Answer from the drawing. Dimensions are ordinates in mm from the lowest x, y and z of the part. Coordinates: 2 decimals unless noted, no trailing zeros. Loops run counter-clockwise (first coordinate to the right, second up) from the corner with the lowest first, then second, coordinate; pieces in that order, holes last. Notation, with made-up numbers: (60.25, 32) -> (92.25, 32) arc R10 ccw to (92.25, 41) -> close; hole circle Ø3 at (6.5, 67). An arc over 180 degrees is marked (long way). Answer as CSV lines item,"result".
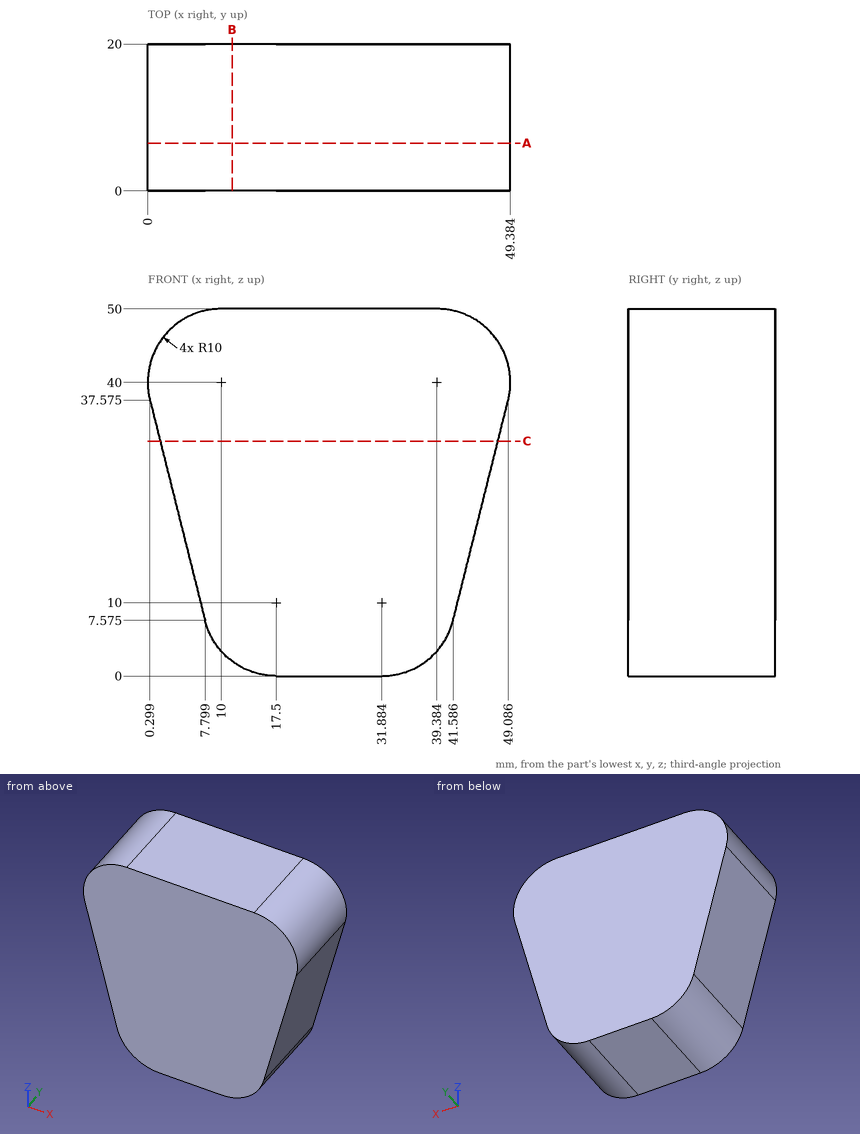
(1) A cutting plane is placed at A-A, the plane y = 6.5. Write down the section's boundary in (x, z) (1 decimal).
Computed values:
outline,"(0.3, 37.6) -> (7.8, 7.6) arc R10 ccw to (17.5, 0) -> (31.9, 0) arc R10 ccw to (41.6, 7.6) -> (49.1, 37.6) arc R10 ccw to (39.4, 50) -> (10, 50) arc R10 ccw to start"
(2) A cutting plane is placed at B-B, the plane x = 11.5. Write down the section's boundary in (y, z), and give its area (3 significant figures).
Computed values:
outline,"(0, 2) -> (20, 2) -> (20, 50) -> (0, 50) -> close"
area,"960 mm2"
(3) Consider line 1 along Z through (x, y) = (17, 1.75); line 2 along X through (y, z) = (11.25, 43) (1 decimal); line 3 along Z through (x, y) = (16, 8.25). Determine where each line is inside the solid, lowest interval first.
Computed values:
line 1,"0.01 to 50"
line 2,"0.5 to 48.9"
line 3,"0.11 to 50"
(4) A cutting plane is placed at C-C, the plane z = 32. Write down the section's boundary in (x, y), and give its area (3 significant figures).
Computed values:
outline,"(1.69, 0) -> (47.69, 0) -> (47.69, 20) -> (1.69, 20) -> close"
area,"920 mm2"
(5) Flat-ended cylindrical pins translate along their axes: pin 1 Ø10 at (x, z) = (39.5, 33.5) entering from -Y; pin 2 Ø2 at (y, z) = (7, 9) entering from +X; pin 3 Ø2 at (y, z) = (14, 31) entering from -X; pin 4 Ø3 at (x, y) = (7, 4.5) entering from +Z. Find the tip coordinate at first contact, or state that the pin passes through.
Computed values:
pin 1,"y = 0"
pin 2,"x = 42.19"
pin 3,"x = 1.69"
pin 4,"z = 49.89"
